Can you work these out from the drawing? Everything is in mm from the part's minimum corner. Coordinates: 2 decimals unless noted, no trailing zeros. Order: outer loops, then holes, each group sorted by start corner. A loop starts at its lowest first (then second) coordinate and runs counter-clockwise, first axis right, second up. Notation, with made-up numbers: M 89.5,32 L 143.5,32 A33 ccw 143.5,63 Z; hole C 29,65.5 d5. An arc over 180 degrees is marked long. Answer as a JSON object with one key per item and string values.
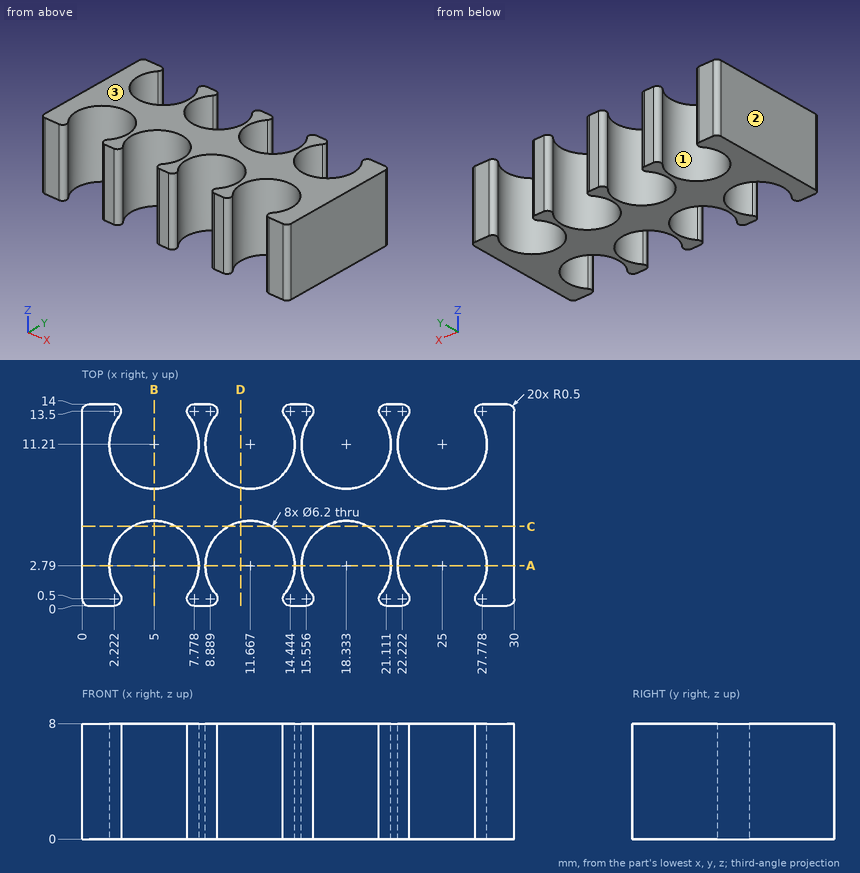
Item 1: If we mould it in two halves opening along X, with no side actions, what happens to the marked faces 1, 2 and 3? For each: pulls with the +X half, pulls with the -X half, needs draft (parallel to the pull), parting line crosses it, or undercut.
Answers follow:
{"face 1": "undercut", "face 2": "pulls with the -X half", "face 3": "needs draft"}
Item 2: I want a section at D-D, the plane x = 11. Write out the boundary of the cut face in (y, z), plus the area to 3 significant figures.
Answers follow:
{"outline": "M 5.82,0 L 8.18,0 L 8.18,8 L 5.82,8 Z", "area": "18.9 mm^2"}
Item 3: I want a section at C-C, the plane y = 5.5. Write out the boundary of the cut face in (x, z) (1 decimal).
Answers follow:
{"outline": "M 0,0 L 3.5,0 L 3.5,8 L 0,8 Z; M 6.5,0 L 10.2,0 L 10.2,8 L 6.5,8 Z; M 13.2,0 L 16.8,0 L 16.8,8 L 13.2,8 Z; M 19.8,0 L 23.5,0 L 23.5,8 L 19.8,8 Z; M 26.5,0 L 30,0 L 30,8 L 26.5,8 Z"}
Item 4: Please list where these lines run through material, in increasing order: line 1 (X direction, y = 11.21, z = 6.25); line 2 (Y direction, x = 7.75, z = 4.25) (1 decimal); line 3 (X direction, y = 8.5, z = 5.5) (1 decimal).
Answers follow:
{"line 1": "x = 0 to 1.9, 8.1 to 8.57, 14.77 to 15.23, 21.43 to 21.9, 28.1 to 30", "line 2": "y = 0 to 1.4, 4.2 to 9.8, 12.6 to 14", "line 3": "x = 0 to 3.5, 6.5 to 10.2, 13.2 to 16.8, 19.8 to 23.5, 26.5 to 30"}
Item 5: I want a section at B-B, the plane x = 5. Write out the boundary of the cut face in (y, z).
Answers follow:
{"outline": "M 5.89,0 L 8.11,0 L 8.11,8 L 5.89,8 Z"}
Item 6: I want a section at A-A, the plane y = 2.79. Write out the boundary of the cut face in (x, z).
Answers follow:
{"outline": "M 0,0 L 1.9,0 L 1.9,8 L 0,8 Z; M 8.1,0 L 8.57,0 L 8.57,8 L 8.1,8 Z; M 14.77,0 L 15.23,0 L 15.23,8 L 14.77,8 Z; M 21.43,0 L 21.9,0 L 21.9,8 L 21.43,8 Z; M 28.1,0 L 30,0 L 30,8 L 28.1,8 Z"}
Item 7: I'm going to push flat-ended pins straight in: pin 1 (2 mm diameter, centred on x = 25.5, y = 12, fed in from -Z); pin 2 (1 mm diameter, centred on x = 25, z = 7, fed in from -Y). Where does each tip first touch, or does it pass through?
Answers follow:
{"pin 1": "passes through", "pin 2": "stops at y = 5.85"}
